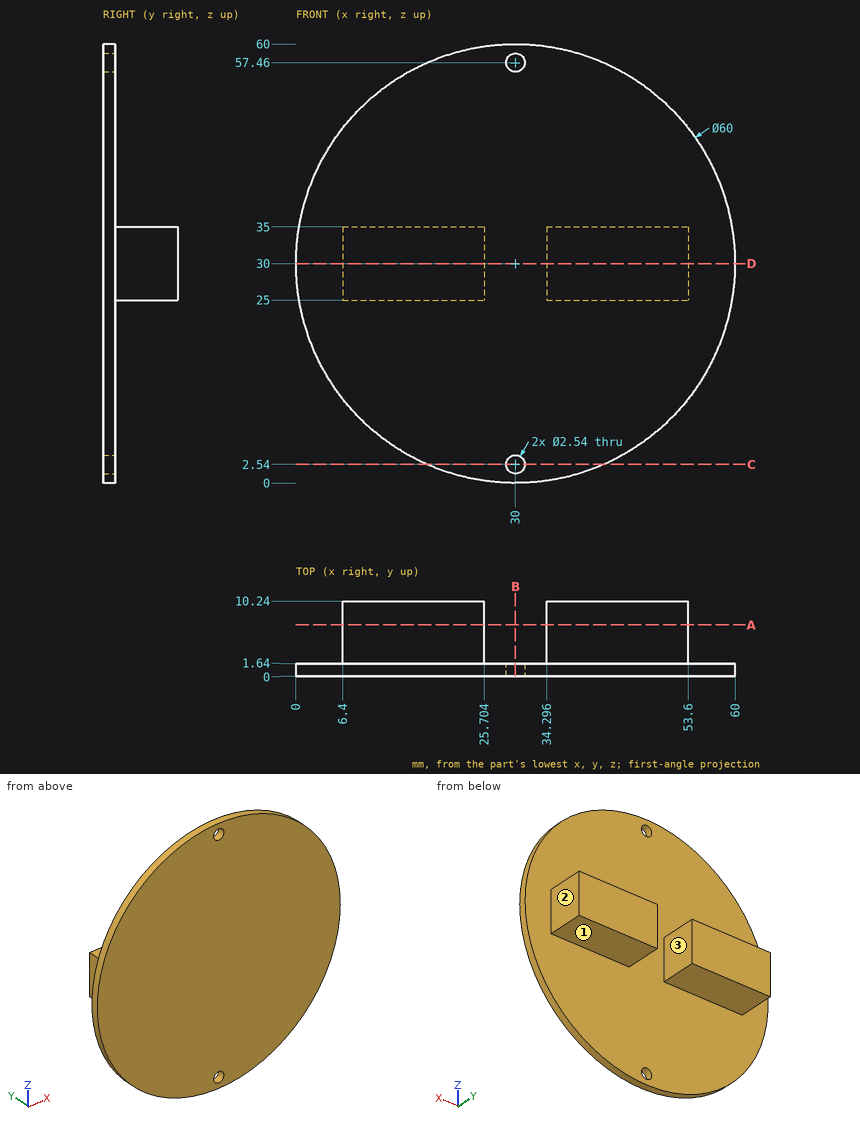
Part print with two shaded views. Sizes in mm from the minimum x, y, z corner. A direction names the side the tool comes from. Give positions to 0.01 mm unless a question says otherwise; leave off trailing zeros. Write each loop counter-clockwise with the first axis right and the second up, starting at its lowest first coordinate (ties: lowest second). Pieces come first, ordered by that corner, then holes.
1) Cut at C-C on z = 2.54. Write the cut outline in (x, y), then the cut area to 3 significant figures.
Resolved:
outline: (17.92, 0) - (28.73, 0) - (28.73, 1.64) - (17.92, 1.64) - close; (31.27, 0) - (42.08, 0) - (42.08, 1.64) - (31.27, 1.64) - close
area: 35.5 mm2
2) Pin check, flat tips, straight feed: pin 1 (2.5 mm diameter, centred on y = 4, z = 31.5, fed in from +X); pin 2 (1.5 mm diameter, centred on x = 30, z = 57.46, fed in from -Y); pin 3 (6 mm diameter, centred on x = 31.5, y = 5.5, fed in from +Z); pin 4 (2.5 mm diameter, centred on x = 42.5, y = 7, fed in from -Z). Stop position of each tip, or through.
Resolved:
pin 1: stops at x = 53.6
pin 2: passes through
pin 3: stops at z = 35
pin 4: stops at z = 25
3) Cut at D-D on z = 30. Write the cut outline in (x, y), then the cut area to 3 significant figures.
Resolved:
outline: (0, 0) - (60, 0) - (60, 1.64) - (53.6, 1.64) - (53.6, 10.24) - (34.3, 10.24) - (34.3, 1.64) - (25.7, 1.64) - (25.7, 10.24) - (6.4, 10.24) - (6.4, 1.64) - (0, 1.64) - close
area: 430 mm2
4) Probe L1, parallel to Z at x = 30, y = 0.7; L2, parallel to Y at x = 35, z = 43; L3, parallel to X at y = 1.35, z = 2.54. List the from-to ranges inside material, lowest first.
Resolved:
L1: z = 0 to 1.27, 3.81 to 56.19, 58.73 to 60
L2: y = 0 to 1.64
L3: x = 17.92 to 28.73, 31.27 to 42.08
5) Cut at A-A on y = 7. Write the cut outline in (x, z).
Resolved:
outline: (6.4, 25) - (25.7, 25) - (25.7, 35) - (6.4, 35) - close; (34.3, 25) - (53.6, 25) - (53.6, 35) - (34.3, 35) - close
6) Cut at B-B on x = 30. Write the cut outline in (y, z), then the cut area to 3 significant figures.
Resolved:
outline: (0, 0) - (1.64, 0) - (1.64, 1.27) - (0, 1.27) - close; (0, 3.81) - (1.64, 3.81) - (1.64, 56.19) - (0, 56.19) - close; (0, 58.73) - (1.64, 58.73) - (1.64, 60) - (0, 60) - close
area: 90.1 mm2
7) Which spindle directions (+Z, -Z, +X, -X, +Y, -Y) get a long thin tool onto all of the face, cutting with end or side? Do the marked faces 1, 2 and 3. Say none if no direction does.
Resolved:
face 1: -Z, +X, -X, +Y
face 2: +Z, -Z, +X, +Y
face 3: +Z, -Z, +Y
